```python
from build123d import *

# Parameters (mm, degrees)
F0_W     = 1018.2218551636
F0_H     = 762.5373601913
F1_DEPTH = 1016
F3_DEPTH = 784.86
F5_DEPTH = 508
F6_W     = 509.1109275818
F6_H     = 508
F7_DEPTH = 543.56


with BuildPart() as f1:
    # F0 (on Front) → F1 (new body)
    with BuildSketch(Plane.XZ):
        with Locations((509.1109275818, 381.2686800957)):
            Rectangle(F0_W, F0_H)
    extrude(amount=F1_DEPTH)

    # F2 (on face) → F3 (cut)
    with BuildSketch(Plane.XY.offset(762.5373601913)):
        Polygon((1018.2218551636, -1016), (0, -508), (0, -1016), align=None)
    extrude(amount=-F3_DEPTH, mode=Mode.SUBTRACT)

    # F4 (on face) → F5 (cut)
    with BuildSketch(Plane.XY.offset(762.5373601913)):
        Polygon((1018.2218551636, -508), (0, -508), (1018.2218551636, -1016), align=None)
    extrude(amount=-F5_DEPTH, mode=Mode.SUBTRACT)

    # F6 (on face) → F7 (cut)
    with BuildSketch(Plane.XZ.offset(508)):
        with Locations((763.6663913727, 508.5373601913)):
            Rectangle(F6_W, F6_H)
    extrude(amount=-F7_DEPTH, mode=Mode.SUBTRACT)


solid = f1.part
```
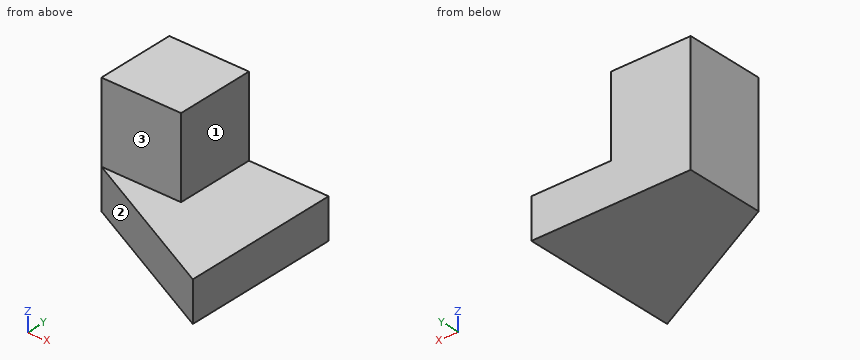
The model under review builds one solid part; all positions refer to its coordinate system, in mm. Face numbers are marked on the shaded views. A direction names the side the tool comes from. Give positions to 0.01 mm unless a question says otherwise; leave off trailing zeros. Write each loop counter-clockwise with the first axis right and the second up, starting at its lowest first coordinate (ties: lowest second). Pieces come first, ordered by that corner, then holes.
(1) For P1, Ø3, axis at x = 779, y = -509.5, coming from the +Z side; P2, Ø12, axis at x = 436, z = 231, coming from the -Y side; P3, Ø4, axis at x = 127.5, z = 286, coming from the -Y side, all flat-tipped, find the tip position at first contact; note any pin that passes through.
(2) Consider section C-C, the plane x = 295.5. Give the boundary of the cut face in (y, z), and give its area (3 significant figures).
(3) Consider section D-D, the plane z = 192. Give the boundary of the cut face in (x, y).
(4) To check wall thickness, follow L1, parallel to Y at x = 386, z = 476.5; L2, parallel to Z at x = 194.5, y = -593; L3, parallel to X at y = -419.5, z = 706.5. State the ranges of each line that lie inside material, in increasing order.
(5) Tool access review of the marked faces 1, 2 and 3: name each direction out of +Z, -Z, +X, -X, +Y, -Y from which nothing blocks a thin tool from reaching the whole face with its end or side.
(6) Consider section A-A, the plane y = -381. Give the boundary of the cut face in (x, z), and give its area (3 significant figures).
(7) Consider section B-B, the plane z = 675.5. Give the boundary of the cut face in (x, y).
Returned:
1. P1: stops at z = 254.54
1. P2: stops at y = -728.52
1. P3: stops at y = -508
2. outline: (-655.43, 0) - (0, 0) - (0, 762.54) - (-508, 762.54) - (-508, 254.54) - (-655.43, 254.54) - close
2. area: 425,000 mm2
3. outline: (0, -508) - (1018.22, -1016) - (1018.22, 0) - (0, 0) - close
4. L1: y = -508 to 0
4. L2: z = 0 to 254.54
4. L3: x = 0 to 509.11
5. face 1: +Z, +X, +Y, -Y
5. face 2: +Z, -Z, -X, -Y
5. face 3: +Z, +X, -X, -Y
6. outline: (0, 0) - (1018.22, 0) - (1018.22, 254.54) - (509.11, 254.54) - (509.11, 762.54) - (0, 762.54) - close
6. area: 518,000 mm2
7. outline: (0, -508) - (509.11, -508) - (509.11, 0) - (0, 0) - close
